Autodesk Inventor part; units mm, degrees
ref_plane "YZ Plane" through (0, 0, 0) normal (1, 0, 0) x (0, 1, 0)
ref_plane "XZ Plane" through (0, 0, 0) normal (0, 1, 0) x (-1, 0, 0)
ref_plane "XY Plane" through (0, 0, 0) normal (0, 0, 1) x (1, 0, 0)
sketch "Sketch1" plane through (0, 0, 0) normal (0, 1, 0) x (-1, 0, 0)
  point P0 (0, 0)
sketch "Sketch2" plane through (0, 0, 0) normal (0, 1, 0) x (-1, 0, 0)
  circle A0 centre (0, 0) radius 31.75
  dimension "d0" = 63.5
extrude "Extrusion1" add sketch "Sketch2" along normal blind 15.875
sketch "Sketch3" plane through (0, 15.875, 0) normal (0, 1, 0) x (1, 0, 0)
  circle A0 centre (0, 0) radius 23.8125
  dimension "d3" = 47.625
extrude "Extrusion2" cut sketch "Sketch3" against normal blind 12.7
chamfer "Chamfer1" distance 0.7937 angle 45 1 edges at (-23.8125, 3.175, 0)
sketch "Sketch4" plane through (0, 3.175, 0) normal (0, 1, 0) x (1, 0, 0)
  circle A0 centre (0, 0) radius 11.1125
  dimension "d12" = 22.225
extrude "Extrusion3" add sketch "Sketch4" along normal blind 15.875
sketch "Sketch5" plane through (0, 19.05, 0) normal (0, 1, 0) x (1, 0, 0)
  circle A0 centre (0, 0) radius 3.175
  dimension "d15" = 6.35
extrude "Extrusion4" add sketch "Sketch5" along normal blind 6.35
chamfer "Chamfer3" distance 3.175 angle 45 1 edges at (-11.1125, 19.05, 0)
sketch "Sketch6" plane through (0, 19.05, 0) normal (0, 1, 0) x (1, 0, 0)
  circle A0 centre (0, 0) radius 7.9375 construction
  circle A1 centre (0, 0) radius 7.9375
  circle A2 centre (0, 7.9375) radius 1.5875
  line L0 (0, 0) -> (0, 7.9375) construction
  circle A3 centre (-6.8741, 3.9688) radius 1.5875
  circle A4 centre (-6.8741, -3.9687) radius 1.5875
  circle A5 centre (0, -7.9375) radius 1.5875
  circle A6 centre (6.8741, -3.9688) radius 1.5875
  circle A7 centre (6.8741, 3.9687) radius 1.5875
  dimension "d21" = 15.875
  dimension "d22" = 3.175
  dimension "d25" = 360
extrude "Extrusion5" cut sketch "Sketch6" against normal through all contours A7 A1 | A1 A7 | A6 A1 | A1 A6 | A2 A1 | A1 A2 | A5 A1 | A1 A5 | A3 A1 | A1 A3 | A4 A1 | A1 A4
sketch "Sketch8" plane through (0, 15.875, 0) normal (0, 1, 0) x (1, 0, 0)
  circle A0 centre (0, 0) radius 23.8125
  circle A1 centre (0, 0) radius 24.6063
  circle A2 centre (0, 0) radius 23.8125
  circle A3 centre (0, 0) radius 31.75
  circle A4 centre (0, 0) radius 3.175
  circle A5 centre (0, 0) radius 30.1625
  dimension "d38" = 0.7937
  dimension "d39" = 47.625
  dimension "d40" = 1.5875
extrude "Extrusion7" cut sketch "Sketch8" against normal blind 12.7 contours A5
fillet "Fillet1" radius 1.5875 2 edges at (-24.6063, 3.175, 0) (-30.1625, 3.175, 0)
sketch "Sketch9" plane through (0, 15.875, 0) normal (0, 1, 0) x (1, 0, 0)
  circle A0 centre (0, 0) radius 19.05
  circle A1 centre (0, 0) radius 25.4
  dimension "d44" = 38.1
  dimension "d45" = 50.8
extrude "Extrusion8" cut sketch "Sketch9" against normal blind 3.175
properties part number "Wheel Mold"
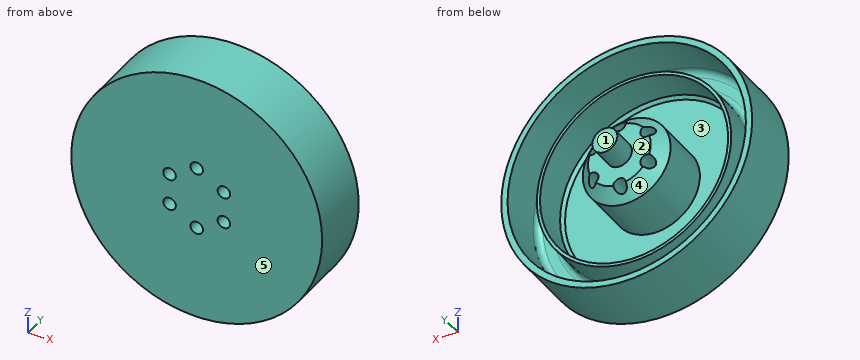
Source: CAD feature listing. Evaluate the final solid. Frame: model axes, mm. Face numbers are marked on the shaded views. A direction names the side the tool comes from. Give positions to 0.01 mm unless a question says otherwise; leave off trailing zeros. Order: outer loops, then holes, each group sorted by start corner. A loop starts at its lowest first (then second) coordinate and runs counter-clockwise, first axis right, second up. Notation, with made-up numbers: (32.25, 71) -> (66.25, 71) arc R9 cw to (66.25, 82) -> close; hole circle Ø4 at (31.25, -30). An arc over 180 degrees is marked (long way). Write item = value, one per line.
Item 1: Ray query, probe 1 along X at (y, z) = (4.75, -14.5); probe 2 along Y at (x, z) = (8, 10) (3 decimals); probe 3 along X at (y, z) = (8.75, -17). Return the intervals inside material, ascending.
Check result:
probe_1 = -28.25 to -26.45, -19.88 to -18.89, 18.89 to 19.88, 26.45 to 28.25
probe_2 = 0 to 3.175
probe_3 = -26.82 to -24.92, -17.79 to -16.67, 16.67 to 17.79, 24.92 to 26.82
Item 2: Mould query, pull axis X, two halves, no side actions, for the marked faces 3, 4 and 5. Classes: +X half, -X half, draft (parallel to the pull), parting line (faces both ways), or undercut.
Check result:
face_3 = undercut
face_4 = parting line
face_5 = draft
Item 3: Contact query for flat-ended pins moving along their axis: pin 1 (5 mm diameter, centred on x = 6.87, z = -3.97, fed in from +Y); pin 2 (5 mm diameter, centred on x = -15, y = 16, fed in from +Z); pin 3 (8 mm diameter, centred on x = -15, z = 19.5, fed in from -Y); pin 4 (1 mm diameter, centred on y = 5, z = -11.5, fed in from +X). Output: stop coordinate, or through.
Check result:
pin_1 = 19.05
pin_2 = 29.18
pin_3 = 0
pin_4 = 29.78
Item 4: Section query D-D (y = 23.75). Output: boundary loops of the cut face in (x, z) (3 decimals).
Check result:
outline = circle Ø6.35 at (0, 0)
Item 5: Section query A-A (y = 10.25). State how many separate pieces and enclosed holes the cut face has, then the cut area to 3 significant figures.
Check result:
separate_pieces = 3
enclosed_holes = 8
area = 770 mm²
Item 6: Set-up query: the marked faces 1 and 2. Return all of +Z, -Z, +X, -X, +Y, -Y with unobstructed straight access to the full face (end or side cutting, diameter ignored); none if empty.
Check result:
face_1 = +Z, -Z, +X, -X, +Y
face_2 = +Y
